Could you check a few things on this model? Use its own coordinates, in mm. Face numbers are marked on the shaded views. A direction names the side the tool comes from. Round coordinates to 2 decimals unless told otherwise and drop trailing zeros. Write each loop counter-clockwise with the first axis right and the second up, starting at its lowest first coordinate (ties: lowest second). Pieces come first, ordered by that corner, then holes. Notation, with made-up numbers: (4.25, 0) -> (45.25, 0) arc R4 cw to (45.25, 6) -> close; hole circle Ø5 at (59, -8.75). An arc over 180 degrees is marked (long way). Answer as CSV lines item,"result". Start each with the question number.
Q1. If we mould it in two halves opening along X, with no side actions, what happens to the marked faces 1, 2, 3 and 4? For each: pulls with the +X half, pulls with the -X half, needs draft (parallel to the pull), parting line crosses it, or undercut.
Q2. For the marked faces 5 and 6, which set-ups out of +Z, -Z, +X, -X, +Y, -Y let a thin tool reach every point of the face, with its end or its side?
Q3. Will these pins go through, and if not, where does the flat tip stop? pin 1 Ø10.5 at (x, z) = (-1.5, 26.5) entering from +Y; pin 2 Ø1.5 at (x, y) = (-9.5, 3) entering from +Z; pin 3 Ø3.5 at (x, z) = (9.5, 17.5) entering from -Y.
Q4. Imagine slicing it at C-C on y = 0.9. Please give me the cut outline in (x, z), and give its area (3 significant figures).
Q5. If I drill on line 1 (Z direction, x = 0, y = 1.5); line 2 (X direction, y = 1.3, z = 18.5); line 3 (X direction, y = 3.95, z = 17), over which ranges is the centre line in solid material (lowest first)? Write a range as [from, to].
Q6. Imagine slicing it at A-A on z = 6.75. Please give me the cut outline in (x, y).
Q7. Imagine slicing it at B-B on x = 0. Please give me the cut outline in (y, z).
Q8. Imagine slicing it at D-D on z = 28.25. Please give me the cut outline in (x, y).
Autodesk Inventor part; units mm, degrees
ref_plane "YZ Plane" through (0, 0, 0) normal (1, 0, 0) x (0, 1, 0)
ref_plane "XZ Plane" through (0, 0, 0) normal (0, 1, 0) x (-1, 0, 0)
ref_plane "XY Plane" through (0, 0, 0) normal (0, 0, 1) x (1, 0, 0)
sketch "Skizze1" plane through (0, 0, 0) normal (0, 1, 0) x (-1, 0, 0)
  line L0 (13.5, 0) -> (-13.5, 0)
  line L1 (-13.5, 0) -> (-13.5, 40)
  line L2 (-13.5, 40) -> (13.5, 40)
  line L3 (13.5, 40) -> (13.5, 0)
  line L4 (0, -12.8) -> (0, 48.8)
  circle A0 centre (0, 6.75) radius 5
  circle A1 centre (0, 28.25) radius 5
  circle A2 centre (0, 28.25) radius 10.75 construction
  circle A3 centre (0, 6.75) radius 10.75 construction
  line L5 (0, 6.75) -> (0, -4) construction
  point P0 (0, 0)
  dimension "d4" = 21.5
  dimension "d0" = 27
  dimension "d1" = 10
  dimension "d2" = 10
  dimension "d3" = 21.5
  dimension "d8" = 4
  dimension "d35" = 40
extrude "Extrusion1" add sketch "Skizze1" along normal blind 6 contours L0 L4 A0 A1 L2 L3 | L0 L1 L2 L4 A1 A0
sketch "Skizze2" plane through (13.5, 0, 0) normal (0, 0, -1) x (-1, 0, 0)
  line L0 (0, 0) -> (27, 0)
  line L1 (0, 6) -> (27, 6)
  line L2 (25.041, 3) -> (0, 3) construction
  line L3 (13.5, 0) -> (13.5, 6) construction
  line L4 (27, 0) -> (27, 6)
  line L5 (0, 0) -> (0, 6)
  point P0 (23, 3)
  point P1 (4, 3)
  dimension "d68" = 9.5
hole "Bohrung1" at (-9.5, 3, 0) at (9.5, 3, 0) direction (0, 0, 1) diameter 2.459 depth 8 tip angle 118
sketch "Skizze5" plane through (0, 6, 0) normal (0, 1, 0) x (1, 0, 0)
  circle A0 centre (0, -28.25) radius 5
  circle A1 centre (0, -28.25) radius 5
  circle A2 centre (0, -6.75) radius 5
  circle A3 centre (0, -6.75) radius 5
  circle A4 centre (0, -28.25) radius 10.55
  circle A5 centre (0, -6.75) radius 10.55
  point P0 (0, 0)
  dimension "d44" = 21.1
extrude "Extrusion2" cut sketch "Skizze5" against normal blind 1
fillet "Fillet2" radius 5 2 edges at (-13.5, 3, 40) (13.5, 3, 40)
sketch "Sketch7" plane through (0, 0, 0) normal (0, -1, 0) x (1, 0, 0)
  arc A0 (13.5, 35) -> (8.5, 40) centre (8.5, 35) ccw construction
  line L0 (-8.5, 40) -> (8.5, 40) construction
  arc A1 (-8.5, 40) -> (-13.5, 35) centre (-8.5, 35) ccw construction
  line L1 (-13.5, 0) -> (-13.5, 35) construction
  line L2 (13.5, 0) -> (-13.5, 0) construction
  line L3 (13.5, 35) -> (13.5, 0) construction
  circle A2 centre (0, 28.25) radius 5 construction
  circle A3 centre (0, 6.75) radius 5 construction
  line L4 (0, 28.25) -> (0, 6.75) construction
  line L5 (-13.5, 0) -> (-13.5, 35) construction
  line L6 (-13.5, 17.5) -> (13.5, 17.5) construction
  line L7 (13.5, 35) -> (13.5, 0) construction
  point P0 (0, 0)
  point P1 (0, 17.5)
  point P2 (-9.5, 17.5)
  point P3 (9.5, 17.5)
  dimension "d66" = 9.5
  dimension "d67" = 9.5
hole "Hole5" at (-9.5, 0, 17.5) at (9.5, 0, 17.5) direction (0, 1, 0) diameter 3.2 depth 8 tip angle 118 counterbore diameter 6 counterbore depth 2
equation "\"d4\" = d3"
properties part number "kicker_base_v2" material "Steel, Carbon"
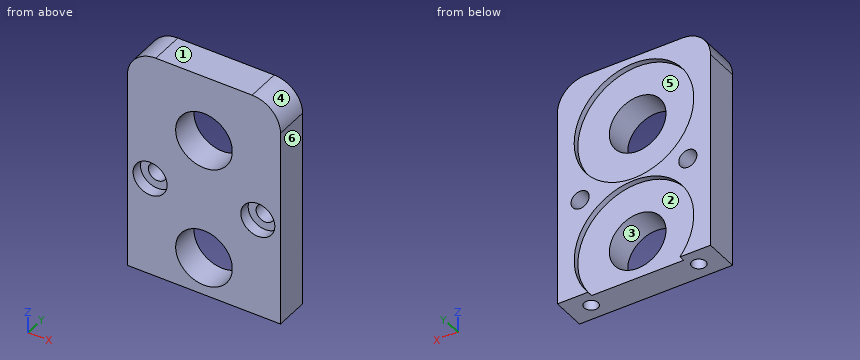
Checks:
1,face 1,"needs draft"
1,face 2,"undercut"
1,face 3,"undercut"
1,face 4,"pulls with the +X half"
2,face 5,"+Y"
2,face 6,"+Z, -Z, +X, +Y, -Y"
3,pin 1,"y = 5"
3,pin 2,"z = 39.99"
3,pin 3,"y = 2"
4,outline,"(-13.5, 0) -> (13.5, 0) -> (13.5, 35) arc R5 ccw to (8.5, 40) -> (-8.5, 40) arc R5 ccw to (-13.5, 35) -> close; hole circle Ø6 at (-9.5, 17.5); hole circle Ø10 at (0, 6.75); hole circle Ø10 at (0, 28.25); hole circle Ø6 at (9.5, 17.5)"
4,area,"856 mm^2"
5,line 1,"[0, 1.75], [11.75, 23.25], [33.25, 40]"
5,line 2,"[-13.5, -12.33], [-6.67, 6.67], [12.33, 13.5]"
5,line 3,"[-13.5, -11.02], [-7.98, 7.98], [11.02, 13.5]"
6,outline,"(-13.5, 0) -> (-5, 0) -> (-5, 5) -> (-10.55, 5) -> (-10.55, 6) -> (-13.5, 6) -> close; (5, 0) -> (13.5, 0) -> (13.5, 6) -> (10.55, 6) -> (10.55, 5) -> (5, 5) -> close; hole circle Ø2.46 at (-9.5, 3); hole circle Ø2.46 at (9.5, 3)"
7,outline,"(0, 0) -> (5, 0) -> (5, 1.75) -> (0, 1.75) -> close; (0, 11.75) -> (5, 11.75) -> (5, 17.3) -> (6, 17.3) -> (6, 17.7) -> (5, 17.7) -> (5, 23.25) -> (0, 23.25) -> close; (0, 33.25) -> (5, 33.25) -> (5, 38.8) -> (6, 38.8) -> (6, 40) -> (0, 40) -> close"
8,outline,"(-13.5, 0) -> (-5, 0) -> (-5, 5) -> (-10.55, 5) -> (-10.55, 6) -> (-13.5, 6) -> close; (5, 0) -> (13.5, 0) -> (13.5, 6) -> (10.55, 6) -> (10.55, 5) -> (5, 5) -> close"
